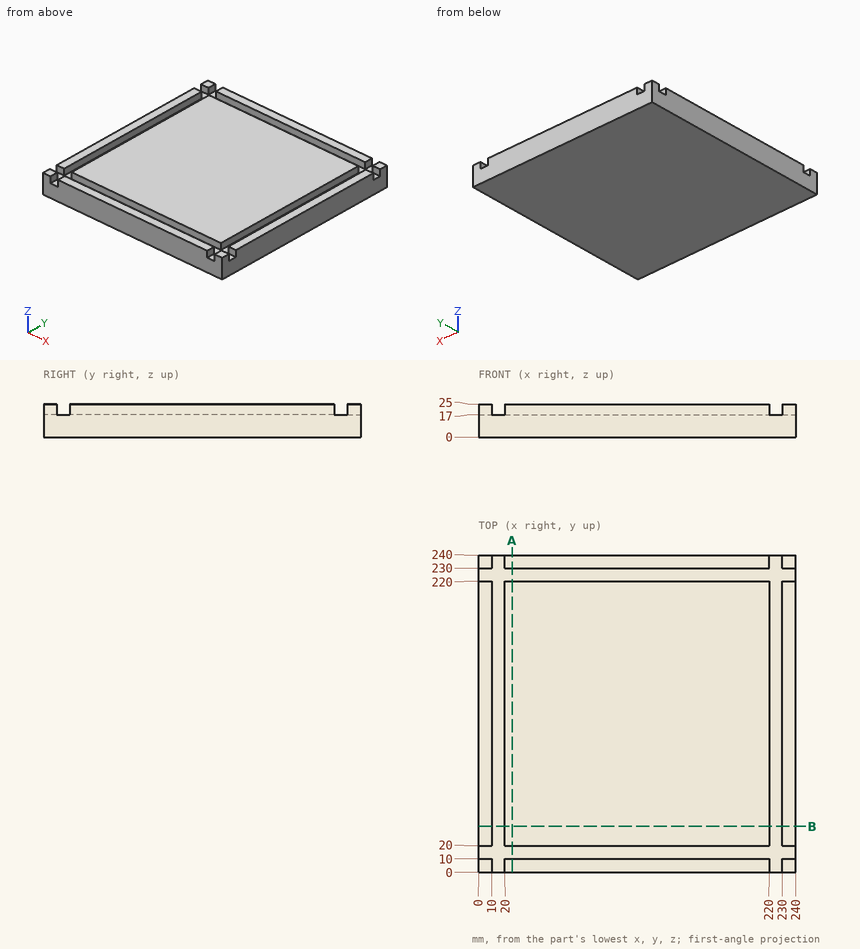
Could you check a few things on this drawing? It's one solid part, dimensions in mm from its lowest x, y, z. Round coordinates to 2 decimals unless told otherwise and drop trailing zeros. Loops run counter-clockwise (first coordinate to the right, second up) from the corner with the lowest first, then second, coordinate; pieces in that order, holes last. Notation, with made-up numbers: M -5.75,10.25 L 52.25,10.25 A21 ccw 52.25,25.25 Z; hole C 60,-34 d11. An arc over 180 degrees is marked long. Write each question's results on one line, items separated by ' | '. Start each with the question number.
(1) I want a section at A-A (x = 25.5). Please give me the cut outline in (y, z), then the cut area to 3 significant figures.
(2) If I drill on probe 1 along Y at (x, z) = (157, 23.25); probe 2 along Z at (x, y) = (134, 12), over which ranges is the centre line in solid material (lowest first)? Write a range as from..to.
Solved:
1) outline: M 0,0 L 240,0 L 240,25 L 230,25 L 230,17 L 220,17 L 220,25 L 20,25 L 20,17 L 10,17 L 10,25 L 0,25 Z | area: 5,840 mm²
2) probe 1: y = 0..10, 20..220, 230..240 | probe 2: z = 0..17
